Geometry check sheet. Reference: the model listing, model coordinates, mm. A direction names the side the tool comes from. Round coordinates to 2 decimals unless told otherwise and drop trailing zeros. Order: outer loops, then holes, each group sorted by start corner. A loop starts at its lowest first (then second) coordinate and runs counter-clockwise, first axis right, second up. Notation, with made-up numbers: (25, 64) - (81, 64) arc R28 cw to (81, 89) - close; hole circle Ø10 at (-13, 18.5). An arc over 180 degrees is marked (long way). Return JSON: item names as keys, results as strings. Group by question number.
Q1. Gauge pin test, flat ends, axial feed: pin 1 Ø2 at (x, z) = (3.5, -16.5) entering from -Y; pin 2 Ø2 at (x, y) = (-1, 7) entering from -Z; pin 3 Ø1 at (x, z) = (2.5, -19) entering from -Y; pin 4 Ø8 at (y, z) = (35, -14.5) entering from -X. Record the tip position at first contact, or that the pin passes through.
Q2. Tool access check on faces 4 (the flat face through (-1, 40.5, -34)), 5 (the cylindrical face through (-4.88, 10.68, -1.08)), 6 (the flat face through (-5, 27.6, -14.5)). Record the directions out of +Z, -Z, +X, -X, +Y, -Y that give a thin tool (end or side, any length) a straight path to the whole face; none if there is none.
Q3. Sectioned sample at B-B, the plane y = 29.5. Record the cut outline in (x, z), then the cut area to 3 significant figures.
Q4. Sectioned sample at A-A, the plane x = 0. Record the cut outline in (y, z).
Q5. Material ranges on line 1 along Y through (x, z) = (2.5, -34.5); line 2 along Z through (x, y) = (2.25, 32.5); line 3 along Y through (x, z) = (-2.75, 0), recorded low to high.
Q6. Sectioned sample at D-D, the plane z = 18. Record the cut outline in (x, y).
Q7. Draft check along Z on faces 1 (the cylindrical face through (-1, 44, -34.2)), 2 (the cylindrical face through (0.07, 28.54, 19.71)), 3 (the flat face through (0, 47.5, 29)). Enter one of: pulls with the +Z half, pulls with the -Z half, needs draft (parallel to the pull), parting line crosses it, or undercut.
Q8. Sectioned sample at C-C, the plane z = -26. Record the cut outline in (x, y).
```python
from build123d import *

# Parameters (mm, degrees)
SKETCH1_R           = 5
BOSS_EXTRUDE1_DEPTH = 23.5
BOSS_EXTRUDE2_DEPTH = 5
SKETCH3_W           = 10
SKETCH3_H           = 15
SKETCH3_R           = 2.5
BOSS_EXTRUDE3_DEPTH = 7


with BuildPart() as part:
    # Sketch1 → Boss-Extrude1 (new body)
    with BuildSketch(Plane(origin=(0, 0, 0), x_dir=(1, 0, 0), z_dir=(0, 1, 0))):
        with Locations(Location((0, 0, 0), (0, 0, 270))):
            Circle(SKETCH1_R)
    extrude(amount=BOSS_EXTRUDE1_DEPTH)

    # Sketch2 → Boss-Extrude2 (add, symmetric)
    with BuildSketch(Plane(origin=(0, 0, 0), x_dir=(0, 0, -1), z_dir=(1, 0, 0))):
        with BuildLine():
            Line((-30.017270029, 47.5), (-27.492699031, 47.5))
            ThreePointArc((-27.492699031, 47.5), (0, 23.75), (27.492699031, 47.5))
            Line((27.492699031, 47.5), (30.017270029, 47.5))
            ThreePointArc((30.017270029, 47.5), (0, 21.25), (-30.017270029, 47.5))
        make_face()
    extrude(amount=BOSS_EXTRUDE2_DEPTH, both=True)

    # Sketch3 → Boss-Extrude3 (add)
    with BuildSketch(Plane(origin=(0, 47.5, 0), x_dir=(1, 0, 0), z_dir=(0, 1, 0))):
        with Locations((0, 34.992699031)):
            Rectangle(SKETCH3_W, SKETCH3_H)
        with Locations(Location((0, 36.492699031, 0), (0, 0, 270))):
            Circle(SKETCH3_R, mode=Mode.SUBTRACT)
    extrude(amount=-BOSS_EXTRUDE3_DEPTH)


solid = part.part
```
Reply:
{
 "1": {"pin 1": "y = 25.52", "pin 2": "z = -5", "pin 3": "y = 27.56", "pin 4": "through"},
 "2": {"face 4": "-Z, +X, -X, -Y", "face 5": "-Y", "face 6": "+Z, -Z, -X, +Y, -Y"},
 "3": {"outline": "(-5, -20.78) - (5, -20.78) - (5, -16.93) - (-5, -16.93) - close; (-5, 16.93) - (5, 16.93) - (5, 20.78) - (-5, 20.78) - close", "area": "77.0 mm^2"},
 "4": {"outline": "(0, -5) - (21.67, -5) arc R30.29 ccw to (40.5, -28.2) - (40.5, -33.99) - (47.5, -33.99) - (47.5, -27.49) arc R27.79 cw to (47.5, 27.49) - (47.5, 30.02) arc R30.29 ccw to (21.67, 5) - (0, 5) - close; (40.5, -42.49) - (47.5, -42.49) - (47.5, -38.99) - (40.5, -38.99) - close"},
 "5": {"line 1": "40.5 to 47.5", "line 2": "-23.56 to -20.24, 20.24 to 23.56", "line 3": "0 to 23.75"},
 "6": {"outline": "(-5, 27.18) - (5, 27.18) - (5, 30.37) - (-5, 30.37) - close"},
 "7": {"face 1": "undercut", "face 2": "pulls with the +Z half", "face 3": "needs draft"},
 "8": {"outline": "(-5, 36) - (5, 36) - (5, 41.73) - (-5, 41.73) - close"}
}
